Design review of the part built by this model. Coordinates are the model's own, in mm. A direction names the side the tool comes from. Round coordinates to 2 decimals unless told otherwise and drop trailing zeros. Order: outer loops, then holes, each group sorted by start corner. A loop starts at its lowest first (then second) coordinate and runs counter-clockwise, first axis right, second up. Notation, with made-up numbers: M 78,36 L 84,36 A16 cw 84,57 Z; hole C 24.5,-17.5 d9. An arc over 180 degrees is marked long. Use a Markdown table: item, result. Add a question column.
(1) For pin 1 (5.5 mm diameter, centred on x = -13, z = 7, fed in from -Y); pin 2 (2 mm diameter, centred on y = 34.2, z = 9, fed in from -X); pin 3 (9 mm diameter, centred on x = 10.5, z = 10, fed in from -Y); pin 4 (1 mm diameter, centred on x = 16, z = 6.5, fed in from -Y), all flat-tipped, find the tip position at first contact; note any pin that passes through.
(2) Machinability: for faces 4 (the face through (-1, 34, 11)), 5 (the face through (-2.52, 35.75, 9.07)), 6 (the face through (30.919, 37.794, 8.874)), 7 (the face through (0.1, -33.2, 8.9)), 8 (the face through (-13, 40.2, 9)), which of the approach directions +Z, -Z, +X, -X, +Y, -Y give a long, thin tool a straight path to every point of the face, cutting with its end or side? Answer none if there is none.
(3) Take a section at A-A (y = 7). Write out the cut boundary in (x, z).
(4) To check wall thickness, follow probe 1 along X at (y, z) = (12.5, 10); probe 2 along Y at (x, z) = (-3, 3.25); probe 3 along X at (y, z) = (31, 4). State the ranges of each line that lie inside material, in increasing order. Write a range as from..to.
(5) The part is to be moulded in two halves that separate along X. For faces 1 (the face through (33.2, 0, 9)), 2 (the face through (0, -41, 0)), 3 (the face through (25.919, -25.794, 8.874)), say which applies: released by +X, released by -X, zero draft, split by the parting line, or undercut.
(6) Take a section at B-B (x = 15). Write out the cut boundary in (y, z), then the cut area to 3 significant figures.
(7) Take a section at D-D (y = 34.2). Write out the cut boundary in (x, z), then the cut area to 3 significant figures.
```python
from build123d import *

# Parameters (mm, degrees)
F0_R     = 4.25
F1_DEPTH = 18
F2_R     = 1.1
F3_DEPTH = 66.401
F2_R_2   = 1.55
F4_DEPTH = 33.2
F5_DEPTH = 29.2


with BuildPart() as f1:
    # F0 (on Top) → F1 (new body)
    with BuildSketch(Plane.XY):
        with BuildLine():
            ThreePointArc((32.761219, -33.2), (33.089542, -31.911773), (33.2, -30.586961))
            Line((33.2, -30.586961), (33.2, 32.2))
            ThreePointArc((33.2, 32.2), (30.856854, 37.856854), (25.2, 40.2))
            Line((25.2, 40.2), (1, 40.2))
            Line((1, 40.2), (1, 33.2))
            Line((1, 33.2), (1, 28.2))
            Line((1, 28.2), (20.2, 28.2))
            ThreePointArc((20.2, 28.2), (25.856854, 25.856854), (28.2, 20.2))
            Line((28.2, 20.2), (28.2, -20.2))
            ThreePointArc((28.2, -20.2), (25.856854, -25.856854), (20.2, -28.2))
            Line((20.2, -28.2), (5.91608, -28.2))
            ThreePointArc((5.91608, -28.2), (5.270583, -28.436237), (4.930066, -29.033333))
            ThreePointArc((4.930066, -29.033333), (0, -33.2), (-4.930066, -29.033333))
            ThreePointArc((-4.930066, -29.033333), (-5.270583, -28.436237), (-5.91608, -28.2))
            Line((-5.91608, -28.2), (-20.2, -28.2))
            ThreePointArc((-20.2, -28.2), (-25.856854, -25.856854), (-28.2, -20.2))
            Line((-28.2, -20.2), (-28.2, 20.2))
            ThreePointArc((-28.2, 20.2), (-25.856854, 25.856854), (-20.2, 28.2))
            Line((-20.2, 28.2), (-1, 28.2))
            Line((-1, 28.2), (-1, 33.2))
            Line((-1, 33.2), (-1, 40.2))
            Line((-1, 40.2), (-25.2, 40.2))
            ThreePointArc((-25.2, 40.2), (-30.856854, 37.856854), (-33.2, 32.2))
            Line((-33.2, 32.2), (-33.2, -30.586961))
            ThreePointArc((-33.2, -30.586961), (-33.089542, -31.911773), (-32.761219, -33.2))
            ThreePointArc((-32.761219, -33.2), (-32.288285, -34.295898), (-31.657565, -35.309233))
            Line((-31.657565, -35.309233), (-6.457565, -69.769474))
            ThreePointArc((-6.457565, -69.769474), (0, -73.047202), (6.457565, -69.769474))
            Line((6.457565, -69.769474), (31.657565, -35.309233))
            ThreePointArc((31.657565, -35.309233), (32.288285, -34.295898), (32.761219, -33.2))
        make_face()
        with Locations((0, -65.9)):
            Circle(F0_R, mode=Mode.SUBTRACT)
    extrude(amount=F1_DEPTH)

    # F2 (on face) → F3 (cut, through all)
    with BuildSketch(Plane(origin=(-33.2, 0, 0), x_dir=(0, -1, 0), z_dir=(-1, 0, 0))):
        with Locations((-34.2, 9)):
            Circle(F2_R)
    extrude(amount=-F3_DEPTH, mode=Mode.SUBTRACT)

    # F2 (on face) → F4 (cut)
    with BuildSketch(Plane(origin=(-33.2, 0, 0), x_dir=(0, -1, 0), z_dir=(-1, 0, 0))):
        with Locations((-34.2, 9)):
            Circle(F2_R_2)
        with Locations((-34.2, 9)):
            Circle(F2_R, mode=Mode.SUBTRACT)
    extrude(amount=-F4_DEPTH, mode=Mode.SUBTRACT)

    # F2 (on face) → F5 (cut)
    with BuildSketch(Plane(origin=(-33.2, 0, 0), x_dir=(0, -1, 0), z_dir=(-1, 0, 0))):
        with BuildLine():
            Line((-32.2, 5.651866), (-32.2, 12.348134))
            ThreePointArc((-32.2, 12.348134), (-38.1, 9), (-32.2, 5.651866))
        make_face()
        with Locations((-34.2, 9)):
            Circle(F2_R_2, mode=Mode.SUBTRACT)
        with BuildLine():
            ThreePointArc((-32.2, 5.651866), (-30.808098, 7.075162), (-30.3, 9))
            ThreePointArc((-30.3, 9), (-30.808098, 10.924838), (-32.2, 12.348134))
            Line((-32.2, 12.348134), (-32.2, 5.651866))
        make_face()
    extrude(amount=-F5_DEPTH, mode=Mode.SUBTRACT)


solid = f1.part
```
Verdict:
| question | item | result |
|---|---|---|
| 1 | pin 1 | stops at y = -64.58 |
| 1 | pin 2 | passes through |
| 1 | pin 3 | stops at y = -70.34 |
| 1 | pin 4 | stops at y = -57.4 |
| 2 | face 4 | +Z, -Z, +Y |
| 2 | face 5 | -X |
| 2 | face 6 | +Z, -Z, +X, +Y |
| 2 | face 7 | +Z, -Z |
| 2 | face 8 | +Z, -Z, +X, -X, +Y |
| 3 | outline | M -33.2,0 L -28.2,0 L -28.2,18 L -33.2,18 Z; M 28.2,0 L 33.2,0 L 33.2,18 L 28.2,18 Z |
| 4 | probe 1 | x = -33.2..-28.2, 28.2..33.2 |
| 4 | probe 2 | y = -72.46..-68.91, -62.89..-32.2, 28.2..40.2 |
| 4 | probe 3 | x = -33.2..-1, 1..33.2 |
| 5 | face 1 | released by +X |
| 5 | face 2 | zero draft |
| 5 | face 3 | undercut |
| 6 | outline | M -58.09,0 L -28.2,0 L -28.2,18 L -58.09,18 Z; M 28.2,0 L 40.2,0 L 40.2,18 L 28.2,18 Z; hole C 34.2,9 d2.2 |
| 6 | area | 750 mm^2 |
| 7 | outline | M -32.95,0 L -1,0 L -1,7.45 L -4,7.45 L -4,5.1 L -32.95,5.1 Z; M -32.95,12.9 L -4,12.9 L -4,10.55 L -1,10.55 L -1,18 L -32.95,18 Z; M 1,0 L 32.95,0 L 32.95,7.9 L 1,7.9 Z; M 1,10.1 L 32.95,10.1 L 32.95,18 L 1,18 Z |
| 7 | area | 845 mm^2 |
